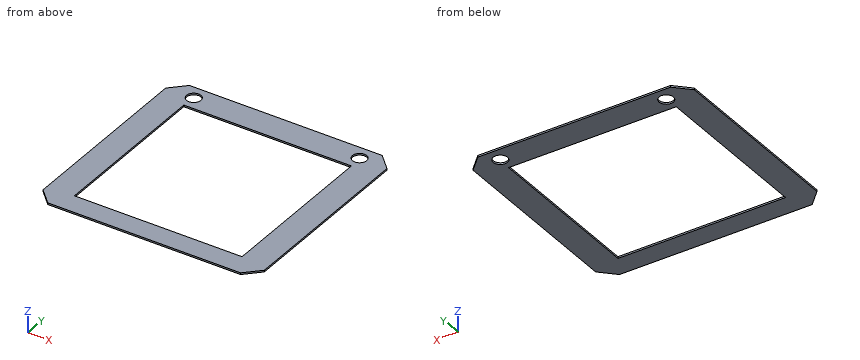
from build123d import *

# Parameters (mm, degrees)
ESQUISSE1_W             = 387
ESQUISSE1_H             = 374
ESQUISSE1_W_2           = 293
ESQUISSE1_H_2           = 289
BOSS_EXTRU_1_DEPTH      = 3
CHANFREIN1_SIZE         = 25
ESQUISSE2_R             = 12.5
ENL_V_MAT_EXTRU_1_DEPTH = 3


with BuildPart() as part:
    # Esquisse1 → Boss.-Extru.1 (new body)
    with BuildSketch(Plane.XY):
        Rectangle(ESQUISSE1_W, ESQUISSE1_H)
        with Locations((0, -5.5)):
            Rectangle(ESQUISSE1_W_2, ESQUISSE1_H_2, mode=Mode.SUBTRACT)
    extrude(amount=BOSS_EXTRU_1_DEPTH)

    # Chanfrein1
    chanfrein1_edges = [part.edges().sort_by_distance(p)[0] for p in [
        (193.5, -187, 1.5),
        (-193.5, -187, 1.5),
        (-193.5, 187, 1.5),
        (193.5, 187, 1.5),
    ]]
    chamfer(chanfrein1_edges, length=CHANFREIN1_SIZE)

    # Esquisse2 → Enlèv. mat.-Extru.1 (cut)
    with BuildSketch(Plane.XY.offset(3)):
        with Locations((145, 163)):
            Circle(ESQUISSE2_R)
        with Locations((-145, 163)):
            Circle(ESQUISSE2_R)
    extrude(amount=-ENL_V_MAT_EXTRU_1_DEPTH, mode=Mode.SUBTRACT)


solid = part.part
Geometry check sheet. Reference: the model listing, model coordinates, mm. Round coordinates to 2 decimals unless told otherwise and drop trailing zeros. Write each loop counter-clockwise with the first axis right and the second up, starting at its lowest first coordinate (ties: lowest second). Pieces come first, ordered by that corner, then holes.
Item 1: Section check B-B (z = 2.4). Record the boundary of the cut face in (x, y), plus the area to 3 significant figures.
Determined:
outline: (-193.5, -162) - (-168.5, -187) - (168.5, -187) - (193.5, -162) - (193.5, 162) - (168.5, 187) - (-168.5, 187) - (-193.5, 162) - close; hole circle Ø25 at (-145, 163); hole (-146.5, -150) - (146.5, -150) - (146.5, 139) - (-146.5, 139) - close; hole circle Ø25 at (145, 163)
area: 57,800 mm2
Item 2: Material ranges on line 1 along Y through (x, z) = (-145, 0.85); line 2 along X through (y, z) = (-117.5, 0.8); line 3 along Y through (x, z) = (-113, 1.7), recorded low to high.
Determined:
line 1: y = -187 to -150, 139 to 150.5, 175.5 to 187
line 2: x = -193.5 to -146.5, 146.5 to 193.5
line 3: y = -187 to -150, 139 to 187
Item 3: Section check A-A (x = 55.5). Record the boundary of the cut face in (y, z), plus the area to 3 significant figures.
Determined:
outline: (-187, 0) - (-150, 0) - (-150, 3) - (-187, 3) - close; (139, 0) - (187, 0) - (187, 3) - (139, 3) - close
area: 255 mm2
